Could you check a few things on this model? Use its own coordinates, in mm. A direction names the side the tool comes from. Coordinates: 2 decimals unless noted, no trailing zeros. Loops run counter-clockwise (first coordinate to the right, second up) from the corner with the lowest first, then second, coordinate; pieces in that order, holes last. Notation, with made-up numbers: (-8, 43.25) - (34, 43.25) arc R18 cw to (34, 63.25) - close; hole circle Ø4 at (7.25, 78.25). An arc over 180 degrees is marked (long way). Put each result on its own line as item: value. Start each with the question number.
```python
from build123d import *

# Parameters (mm, degrees)
SKETCH3_R          = 2
CUT_EXTRUDE1_DEPTH = 10
CUT_EXTRUDE2_DEPTH = 2


with BuildPart() as part:
    # Sketch2 → Revolve1 (revolve)
    with BuildSketch(Plane.XY, mode=Mode.PRIVATE) as revolve1_sk:
        Polygon((-54.3, 0), (-54.3, 5), (-52.3, 5), (-52.3, 7.5), (-46.3, 7.5), (-46.3, 25.4), (-14.8, 25.4), (-14.8, 26.15), (0, 26.15), (0, 4), (35, 4), (35, 0), align=None)
    revolve(revolve1_sk.sketch.rotate(Axis((-163.925373134, 0, 0), (1, 0, 0)), 180), axis=Axis((-163.925373134, 0, 0), (1, 0, 0)))

    # Sketch3 → Cut-Extrude1 (cut)
    with BuildSketch(Plane(origin=(0, 0, 0), x_dir=(0, 0, -1), z_dir=(1, 0, 0))):
        with Locations(Location((-15.556349186, -15.556349186, 0), (0, 0, 90))):
            Circle(SKETCH3_R)
        with Locations(Location((-15.556349186, 15.556349186, 0), (0, 0, 90))):
            Circle(SKETCH3_R)
        with Locations(Location((15.556349186, 15.556349186, 0), (0, 0, 90))):
            Circle(SKETCH3_R)
        with Locations(Location((15.556349186, -15.556349186, 0), (0, 0, 90))):
            Circle(SKETCH3_R)
    extrude(amount=-CUT_EXTRUDE1_DEPTH, mode=Mode.SUBTRACT)

    # Sketch5 → Cut-Extrude2 (cut)
    with BuildSketch(Plane(origin=(0, -4, 0), x_dir=(-1, 0, 0), z_dir=(0, -1, 0))):
        with BuildLine():
            Line((-12.5, -1.5), (-17.5, -1.5))
            ThreePointArc((-17.5, -1.5), (-19, 0), (-17.5, 1.5))
            Line((-17.5, 1.5), (-12.5, 1.5))
            ThreePointArc((-12.5, 1.5), (-11, 0), (-12.5, -1.5))
        make_face()
    extrude(amount=-CUT_EXTRUDE2_DEPTH, mode=Mode.SUBTRACT)


solid = part.part
```
(1) I need wall thicknesses on L1, parallel to X at y = 3.5, z = -9.5; L2, parallel to Y at x = -0.5, z = 16; L3, parallel to Z at x = -1.5, y = -14. Which ranges of each line are inside material? Lowest first, please. Write a range as [from, to].
(2) I want a section at D-D on z = 10. List the corners of the cut face in (x, y) for me.
(3) I want a section at C-C on x = -24.5. List the corners of the cut face in (y, z) for me.
(4) Which directions (+Z, -Z, +X, -X, +Y, -Y) give clear straight access to the entire face, cutting with the end or side of a thin tool? Please do faces 1 (the cylindrical face through (-4.93, -17.554, 15.644)), 2 (the cylindrical face through (-53, 5, 0)), 3 (the flat face through (15, -2, 0)).
(5) If we mould it in two halves opening along Z, with no side actions, what happens to faces 4 (the flat face through (35, 0, 0)), 5 (the flat face through (-10, 16, -16)), 6 (the cylindrical face through (-7.3, -12.07, 23.2))? For each: pulls with the +Z half, pulls with the -Z half, needs draft (parallel to the pull), parting line crosses it, or undercut.
(6) For pin 1 Ø8 at (y, z) = (-20, -6) entering from -X; pin 2 Ø1.5 at (x, z) = (13, -0.5) entering from -Y; pin 3 Ø5 at (x, y) = (-19.5, -10) entering from +Z, each with a flat end and sliding along its axis, tell me the tip position at first contact or that it passes through.
(7) I want a section at A-A on y = 0. List the corners of the cut face in (x, z) for me.
(8) I want a section at B-B on z = 0. List the corners of the cut face in (x, y) for me, and give its area (3 significant figures).
Answer sheet:
1. L1: x = [-46.3, 0]
1. L2: y = [-20.68, -17.51], [-13.61, 13.61], [17.51, 20.68]
1. L3: z = [-22.09, -16.81], [-14.3, 14.3], [16.81, 22.09]
2. outline: (-46.3, -23.35) - (-14.8, -23.35) - (-14.8, -24.16) - (0, -24.16) - (0, 24.16) - (-14.8, 24.16) - (-14.8, 23.35) - (-46.3, 23.35) - close
3. outline: circle Ø50.8 at (0, 0)
4. face 1: +X
4. face 2: -X
4. face 3: -Y
5. face 4: needs draft
5. face 5: undercut
5. face 6: parting line crosses it
6. pin 1: stops at x = -46.3
6. pin 2: stops at y = -2
6. pin 3: stops at z = 24.27
7. outline: (-54.3, -5) - (-52.3, -5) - (-52.3, -7.5) - (-46.3, -7.5) - (-46.3, -25.4) - (-14.8, -25.4) - (-14.8, -26.15) - (0, -26.15) - (0, -4) - (35, -4) - (35, 4) - (0, 4) - (0, 26.15) - (-14.8, 26.15) - (-14.8, 25.4) - (-46.3, 25.4) - (-46.3, 7.5) - (-52.3, 7.5) - (-52.3, 5) - (-54.3, 5) - close
8. outline: (-54.3, -5) - (-52.3, -5) - (-52.3, -7.5) - (-46.3, -7.5) - (-46.3, -25.4) - (-14.8, -25.4) - (-14.8, -26.15) - (0, -26.15) - (0, -4) - (11, -4) - (11, -2) - (19, -2) - (19, -4) - (35, -4) - (35, 4) - (0, 4) - (0, 26.15) - (-14.8, 26.15) - (-14.8, 25.4) - (-46.3, 25.4) - (-46.3, 7.5) - (-52.3, 7.5) - (-52.3, 5) - (-54.3, 5) - close
8. area: 2,750 mm^2
